```python
from build123d import *

# Parameters (mm, degrees)
BOSS_EXTRUDE1_DEPTH = 115
SKETCH1_3_W         = 3
SKETCH1_3_H         = 6
CUT_EXTRUDE1_DEPTH  = 10


with BuildPart() as part:
    # Sketch1 → Boss-Extrude1 (new body)
    with BuildSketch(Plane.XY):
        with BuildLine():
            ThreePointArc((1.5, 4.520111309), (0, 4.7625), (-1.5, 4.520111309))
            Line((-1.5, 4.520111309), (-1.5, 1.7625))
            Line((-1.5, 1.7625), (1.5, 1.7625))
            Line((1.5, 1.7625), (1.5, 4.520111309))
        make_face()
        with BuildLine():
            Line((-1.5, 1.7625), (-1.5, 4.520111309))
            ThreePointArc((-1.5, 4.520111309), (-2.787261761, -3.861680738), (4.7625, 0))
            ThreePointArc((4.7625, 0), (3.861680738, 2.787261761), (1.5, 4.520111309))
            Line((1.5, 4.520111309), (1.5, 1.7625))
            Line((1.5, 1.7625), (-1.5, 1.7625))
        make_face()
    extrude(amount=BOSS_EXTRUDE1_DEPTH)

    # Sketch1_3 → Cut-Extrude1 (cut)
    with BuildSketch(Plane.XY):
        with Locations((0, 4.7625)):
            Rectangle(SKETCH1_3_W, SKETCH1_3_H)
    extrude(amount=CUT_EXTRUDE1_DEPTH, mode=Mode.SUBTRACT)


solid = part.part
```
Part model, mm, in its own coordinate system. A direction names the side the tool comes from. Give positions to 0.01 mm unless a question says otherwise; leave off trailing zeros. Order: outer loops, then holes, each group sorted by start corner. A loop starts at its lowest first (then second) coordinate and runs counter-clockwise, first axis right, second up. Notation, with made-up numbers: M 42,-6 L 72,-6 A33 cw 72,28 Z; hole C 74.25,24.25 d2. An arc over 180 degrees is marked long. Use a Markdown table: item, result. Add a question column.
(1) Probe line 1 along Z through (x, y) = (-0.75, 2.75); line 2 along X through (y, z) = (-0.25, 35.5); line 3 along X through (y, z) = (2.5, 8). List the from-to ranges inside material, lowest first. Write a range as [from, to].
(2) Drop flat-ended pins along their axis: P1, Ø1, axis at y = 1, z = 61, coming from the +X side; P2, Ø2, axis at y = 3.5, z = 5, coming from the +X side; P3, Ø3, axis at x = 2, z = 41.5, coming from the -Y side. Give the stop position or say it passes through.
(3) 3-axis set-ups, long thin cutter, end or side, ignore diameter. For faces 1 (the face through (1.5, 3, 5)), 2 (the face through (0, 0, 115)): which of +Z, -Z, +X, -X, +Y, -Y reach the whole face in a straight line?
(4) Saw through at C-C, the plane z = 65. Give the cut face in (x, y) (1 decimal), and give its area (3 significant figures).
(5) Saw through at B-B, the plane x = 0. Give the cut face in (y, z), and give its area (3 significant figures).
(6) Saw through at D-D, the plane y = -3. Give the cut face in (x, z), and give its area (3 significant figures).
(7) Saw through at A-A, the plane y = 3. Give the cut face in (x, z).
Answer key:
| question | item | result |
|---|---|---|
| 1 | line 1 | [10, 115] |
| 1 | line 2 | [-4.76, 4.76] |
| 1 | line 3 | [-4.05, -1.5], [1.5, 4.05] |
| 2 | P1 | x = 4.74 |
| 2 | P2 | x = 4.05 |
| 2 | P3 | y = -4.74 |
| 3 | face 1 | -Z, +Y |
| 3 | face 2 | +Z, +X, -X, +Y, -Y |
| 4 | outline | C 0,0 d9.5 |
| 4 | area | 71.3 mm^2 |
| 5 | outline | M -4.76,0 L 1.76,0 L 1.76,10 L 4.76,10 L 4.76,115 L -4.76,115 Z |
| 5 | area | 1,070 mm^2 |
| 6 | outline | M -3.7,0 L 3.7,0 L 3.7,115 L -3.7,115 Z |
| 6 | area | 851 mm^2 |
| 7 | outline | M -3.7,0 L -1.5,0 L -1.5,10 L 1.5,10 L 1.5,0 L 3.7,0 L 3.7,115 L -3.7,115 Z |
